```python
from build123d import *

# Parameters (mm, degrees)
F0_R     = 29.9274598154
F1_DEPTH = 75.92757
F2_R     = 27.9824251374
F3_DEPTH = 42.964930072
F4_R     = 6.0972524399
F5_DEPTH = 31.6609
F6_DEPTH = 6.63492


# Not quite as in the source:
# - a feature names something its author has since deleted; it is built from what else it names


with BuildPart() as f1:
    # F0 (on Front) → F1 (new body)
    with BuildSketch(Plane.XZ):
        Circle(F0_R)
    extrude(amount=F1_DEPTH)

    # F2
    f2_edges = [f1.edges().sort_by_distance(p)[0] for p in [
        (-29.92746, -75.92757, 0),
    ]]
    fillet(f2_edges, radius=F2_R)

    # F3 (add): a face of the model
    f3_faces = [f1.faces().sort_by_distance(p)[0] for p in [
        (0, 0, 0),
    ]]
    extrude(f3_faces, amount=F3_DEPTH)

    # F4 (on Top) → F5 (join)
    with BuildSketch(Plane.XY):
        with Locations((0, -48.1517650187)):
            Circle(F4_R)
    extrude(amount=F5_DEPTH)

    # F6 (add): a face of the model
    f6_faces = [f1.faces().sort_by_distance(p)[0] for p in [
        (0, -48.1517650187, 31.6609),
    ]]
    extrude(f6_faces, amount=-F6_DEPTH)


solid = f1.part
```
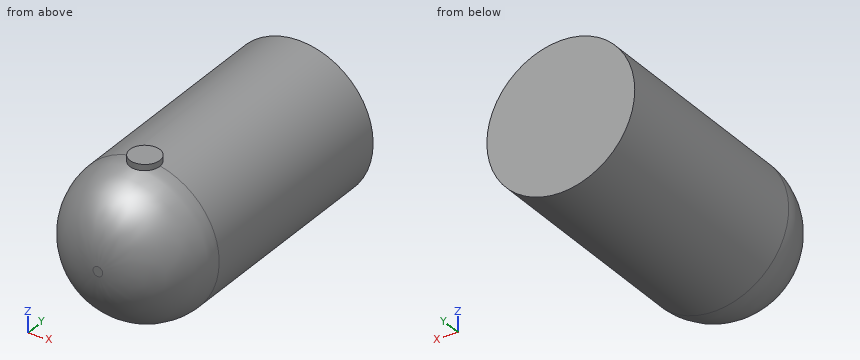
The listing builds one solid part. Answer for the finished solid, in the listing's coordinates (mm). Coordinates: 2 decimals unless noted, no trailing zeros. Write each loop counter-clockwise with the first axis right and the second up, starting at its lowest first coordinate (ties: lowest second). Pieces come first, ordered by that corner, then holes.
Q1. Given P1, Ø10, axis at y = 18.5, z = 17, coming from the -X side; P2, Ø8, axis at x = 19, y = 10.5, coming from the +Z side; P3, Ø12, axis at y = 1.5, z = 6, coming from the -X side; P4, Ø10, axis at y = 1, z = 21, coming from the -X side, each flat-ended and moving along its own axis, determine where each tip first touches the part or whether it passes through.
Returned:
P1: stops at x = -27.42
P2: stops at z = 25.9
P3: stops at x = -29.93
P4: stops at x = -25.29
Q2. Find the intervals of material crossed by line 1 along Y through (x, z) = (-2.5, 1.5); line 2 along Z through (x, y) = (11, -21.5); line 3 along Y through (x, z) = (-3.5, 18), in increasing order.
Returned:
line 1: y = -75.91 to 42.96
line 2: z = -27.83 to 27.83
line 3: y = -70.62 to 42.96
Q3. Section A-A, the plane y = -1 is taken. Write down the section's boundary in (x, z).
Returned:
outline: circle Ø59.85 at (0, 0)
